```python
from build123d import *

# Parameters (mm, degrees)
SKETCH1_W          = 431.8
SKETCH1_H          = 368.3
BASE_FLANGE1_DEPTH = 12.7
EDGE_FLANGE1_DEPTH = 431.8
EDGE_FLANGE2_DEPTH = 431.8
EDGE_FLANGE3_DEPTH = 368.3
EDGE_FLANGE4_DEPTH = 368.3


# Sheet-metal steps are written as plain solids
with BuildPart() as part:
    # Sketch1 → Base-Flange1 (new body)
    with BuildSketch(Plane.XY):
        Rectangle(SKETCH1_W, SKETCH1_H)
    extrude(amount=BASE_FLANGE1_DEPTH)

    # Edge-Flange1 section (across the edge) → Edge-Flange1 (add)
    with BuildSketch(Plane(origin=(215.9, 185.42, 12.7), x_dir=(0, -1, 0), z_dir=(-1, 0, 0))):
        with BuildLine():
            Line((-12.7, 1.27), (-12.7, 4.7244))
            Line((-12.7, 4.7244), (0, 4.7244))
            Line((0, 4.7244), (0, 1.27))
            ThreePointArc((0, 1.27), (0.371974388, 0.371974388), (1.27, 0))
            Line((1.27, 0), (1.27, -12.7))
            ThreePointArc((1.27, -12.7), (-8.608281733, -8.608281733), (-12.7, 1.27))
        make_face()
    extrude(amount=EDGE_FLANGE1_DEPTH)

    # Edge-Flange2 section (across the edge) → Edge-Flange2 (add)
    with BuildSketch(Plane(origin=(-215.9, -185.42, 12.7), x_dir=(0, 1, 0), z_dir=(1, 0, 0))):
        with BuildLine():
            Line((-12.7, 1.27), (-12.7, 4.7244))
            Line((-12.7, 4.7244), (0, 4.7244))
            Line((0, 4.7244), (0, 1.27))
            ThreePointArc((0, 1.27), (0.371974388, 0.371974388), (1.27, 0))
            Line((1.27, 0), (1.27, -12.7))
            ThreePointArc((1.27, -12.7), (-8.608281733, -8.608281733), (-12.7, 1.27))
        make_face()
    extrude(amount=EDGE_FLANGE2_DEPTH)

    # Edge-Flange3 section (across the edge) → Edge-Flange3 (add)
    with BuildSketch(Plane(origin=(217.17, -184.15, 12.7), x_dir=(-1, 0, 0), z_dir=(0, 1, 0))):
        with BuildLine():
            Line((-12.7, 1.27), (-12.7, 4.7244))
            Line((-12.7, 4.7244), (0, 4.7244))
            Line((0, 4.7244), (0, 1.27))
            ThreePointArc((0, 1.27), (0.371974388, 0.371974388), (1.27, 0))
            Line((1.27, 0), (1.27, -12.7))
            ThreePointArc((1.27, -12.7), (-8.608281733, -8.608281733), (-12.7, 1.27))
        make_face()
    extrude(amount=EDGE_FLANGE3_DEPTH)

    # Edge-Flange4 section (across the edge) → Edge-Flange4 (add)
    with BuildSketch(Plane(origin=(-217.17, 184.15, 12.7), x_dir=(1, 0, 0), z_dir=(0, -1, 0))):
        with BuildLine():
            Line((-12.7, 1.27), (-12.7, 4.7244))
            Line((-12.7, 4.7244), (0, 4.7244))
            Line((0, 4.7244), (0, 1.27))
            ThreePointArc((0, 1.27), (0.371974388, 0.371974388), (1.27, 0))
            Line((1.27, 0), (1.27, -12.7))
            ThreePointArc((1.27, -12.7), (-8.608281733, -8.608281733), (-12.7, 1.27))
        make_face()
    extrude(amount=EDGE_FLANGE4_DEPTH)


solid = part.part
```
Read the model definition and answer for the solid it produces. Units are mm, in the model's axes. A direction names the side the tool comes from. Round coordinates to 2 decimals unless told otherwise and drop trailing zeros. Write each loop counter-clockwise with the first axis right and the second up, starting at its lowest first coordinate (ties: lowest second). Pieces come first, ordered by that corner, then holes. Notation, with made-up numbers: M -5,7.5 L 42,7.5 A4 cw 42,12.5 Z; hole C 31.25,-31 d11. An arc over 180 degrees is marked long. One line per item, written item: value.
Q1. Which of the six approach directions +Z, -Z, +X, -X, +Y, -Y give full straight-line access (tool end or side, diameter ignored) to faces 5 (the flat face through (-215.9, -191, 9)), 6 (the flat face through (215.9, 191, 9)), 7 (the flat face through (223, -184.15, 9)), 8 (the flat face through (-215.9, 191, 9))?
Data:
face 5: +Z, -Z, -X, -Y
face 6: +Z, -Z, +X, +Y
face 7: +Z, -Z, +X, -Y
face 8: +Z, -Z, -X, +Y
Q2. Find section A-A on x = 37. Write down the section's boundary in (y, z), plus the area to 3 significant figures.
Data:
outline: M -198.12,13.97 A13.97 ccw -184.15,0 L 184.15,0 A13.97 ccw 198.12,13.97 L 198.12,17.42 L 185.42,17.42 L 185.42,13.97 A1.27 cw 184.15,12.7 L -184.15,12.7 A1.27 cw -185.42,13.97 L -185.42,17.42 L -198.12,17.42 Z
area: 5,070 mm2
Q3. Straight lines are drawn through the part: line 1 (Y direction, x = -190, z = 15.5); line 2 (X direction, y = -104.5, z = 16.5); line 3 (Z direction, x = 66, y = -51). For each, find the intervals that lie inside material, in ascending order. Write a range as [from, to].
Data:
line 1: [-198.12, -185.42], [185.42, 198.12]
line 2: [-229.87, -217.17], [217.17, 229.87]
line 3: [0, 12.7]
Q4. Flat-ended cylindrical pins translate along their axes: pin 1 Ø1.5 at (x, z) = (-170.5, 11.5) entering from +Y; pin 2 Ø7 at (x, z) = (-224.5, 13) entering from -Y; pin 3 Ø7 at (y, z) = (194.5, 5.5) entering from -X. Find the tip coordinate at first contact, or state that the pin passes through.
Data:
pin 1: y = 198.01
pin 2: y = -184.15
pin 3: x = -215.9
Q5. For a pull along X with two mould halves and no side action, classify faces 1 (the cylindrical face through (-3.023, -193.919, 3.984)), 2 (the flat face through (215.9, -191, 9)), 3 (the cylindrical face through (-225.669, 2.578, 3.984)), 4 (the flat face through (-3, 3, 12.7)) as +X half, -X half, draft (parallel to the pull), parting line (faces both ways), or undercut.
Data:
face 1: draft
face 2: +X half
face 3: -X half
face 4: undercut
Q6. Find section B-B on y = -81. Write down the section's boundary in (x, z), plus the area to 3 significant figures.
Data:
outline: M -229.87,13.97 A13.97 ccw -215.9,0 L 215.9,0 A13.97 ccw 229.87,13.97 L 229.87,17.42 L 217.17,17.42 L 217.17,13.97 A1.27 cw 215.9,12.7 L -215.9,12.7 A1.27 cw -217.17,13.97 L -217.17,17.42 L -229.87,17.42 Z
area: 5,880 mm2
